```python
from build123d import *

# Parameters (mm, degrees)
SKETCH1_W           = 86.9
SKETCH1_H           = 86.9
BOSS_EXTRUDE1_DEPTH = 2
SKETCH2_R           = 1.65
CUT_EXTRUDE3_DEPTH  = 123.911431527
SKETCH3_W           = 18
SKETCH3_H           = 17
BOSS_EXTRUDE2_DEPTH = 1
SKETCH4_W           = 13
SKETCH4_H           = 14
CUT_EXTRUDE4_DEPTH  = 1
SKETCH5_R           = 15
CUT_EXTRUDE5_DEPTH  = 2


with BuildPart() as part:
    # Sketch1 → Boss-Extrude1 (new body)
    with BuildSketch(Plane(origin=(0, 0, 0), x_dir=(0, 1, 0), z_dir=(0, 0, 1))):
        with Locations((43.45, 43.45)):
            Rectangle(SKETCH1_W, SKETCH1_H)
    extrude(amount=BOSS_EXTRUDE1_DEPTH)

    # Sketch2 → Cut-Extrude3 (cut, through all)
    with BuildSketch(Plane.XY.offset(2)):
        with Locations((-84.05, 2.85)):
            Circle(SKETCH2_R)
        with Locations((-2.85, 2.85)):
            Circle(SKETCH2_R)
        with Locations((-2.85, 84.05)):
            Circle(SKETCH2_R)
        with Locations((-84.05, 84.05)):
            Circle(SKETCH2_R)
    extrude(amount=-CUT_EXTRUDE3_DEPTH, mode=Mode.SUBTRACT)

    # Sketch3 → Boss-Extrude2 (add)
    with BuildSketch(Plane.XY.offset(2)):
        with Locations((-63.4, 23.5)):
            Rectangle(SKETCH3_W, SKETCH3_H)
    extrude(amount=BOSS_EXTRUDE2_DEPTH)

    # Sketch4 → Cut-Extrude4 (cut)
    with BuildSketch(Plane.XY.offset(3)):
        with Locations((-63.4, 23.5)):
            Rectangle(SKETCH4_W, SKETCH4_H)
    extrude(amount=-CUT_EXTRUDE4_DEPTH, mode=Mode.SUBTRACT)

    # Sketch5 → Cut-Extrude5 (cut)
    with BuildSketch(Plane.XY.offset(2)):
        with Locations((-63.45, 63.45)):
            Circle(SKETCH5_R)
        with Locations((-23.45, 63.45)):
            Circle(SKETCH5_R)
        with Locations((-23.45, 23.45)):
            Circle(SKETCH5_R)
    extrude(amount=-CUT_EXTRUDE5_DEPTH, mode=Mode.SUBTRACT)


solid = part.part
```
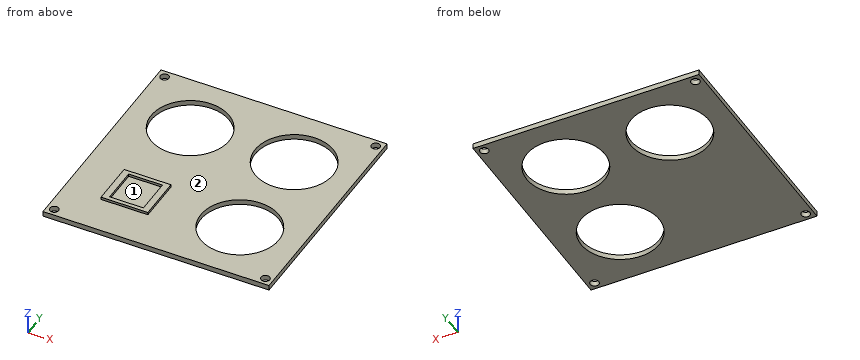
Check sheet for the modelled part. Datum: model origin and axes. Units: mm. Face numbers are marked on the shaded views. Give positions to 0.01 mm unless a question says otherwise; leave off trailing zeros. Order: outer loops, then holes, each group sorted by start corner. A loop starts at its lowest first (then second) coordinate and runs counter-clockwise, first axis right, second up. Notation, with made-up numbers: M -10,2.25 L 36,2.25 A31 cw 36,35.25 Z; hole C -32.5,-17 d6. An arc over 180 degrees is marked long. Answer in a Markdown table with one row per item. Add a question column.
Q1. Sectioned sample at D-D, the plane z = 2.5. Record the boundary of the cut face in (x, y), and give its area (3 significant figures).
Q2. Sectioned sample at B-B, the plane x = -2.85. Record the boundary of the cut face in (y, z).
Q3. Sectioned sample at A-A, the plane y = 84.05. Record the boundary of the cut face in (x, z).
Q4. Sectioned sample at C-C, the plane y = 23.45. Record the boundary of the cut face in (x, z), and give its area (3 significant figures).
Q5. Release check for a two-part mould opening along Y. For the marked faces 1 and 2 record: released by +Y, released by -Y, zero draft, split by the parting line, or undercut.
Q6. Thickness scan on L1, parallel to X at y = 84.05, z = 1.2; L2, parallel to Y at x = -84.05, z = 1.1; L3, parallel to X at y = 23, z = 1.5. Record the ranges inside material, lowest first.
Q7. Gauge pin test, flat ends, axial feed: pin 1 Ø2.5 at (x, y) = (-84.05, 84.05) entering from -Z; pin 2 Ø0.8 at (y, z) = (20, 2.5) entering from +X; pin 3 Ø0.5 at (x, z) = (-66, 2.5) entering from +Y; pin 4 Ø4 at (x, y) = (-60, 20) entering from +Z. Record the tip position at first contact, or that the pin passes through.
Verdict:
| question | item | result |
|---|---|---|
| 1 | outline | M -72.4,15 L -54.4,15 L -54.4,32 L -72.4,32 Z; hole M -69.9,16.5 L -56.9,16.5 L -56.9,30.5 L -69.9,30.5 Z |
| 1 | area | 124 mm² |
| 2 | outline | M 0,0 L 1.2,0 L 1.2,2 L 0,2 Z; M 4.5,0 L 82.4,0 L 82.4,2 L 4.5,2 Z; M 85.7,0 L 86.9,0 L 86.9,2 L 85.7,2 Z |
| 3 | outline | M -86.9,0 L -85.7,0 L -85.7,2 L -86.9,2 Z; M -82.4,0 L -4.5,0 L -4.5,2 L -82.4,2 Z; M -1.2,0 L 0,0 L 0,2 L -1.2,2 Z |
| 4 | outline | M -86.9,0 L -38.45,0 L -38.45,2 L -54.4,2 L -54.4,3 L -56.9,3 L -56.9,2 L -69.9,2 L -69.9,3 L -72.4,3 L -72.4,2 L -86.9,2 Z; M -8.45,0 L 0,0 L 0,2 L -8.45,2 Z |
| 4 | area | 119 mm² |
| 5 | face 1 | undercut |
| 5 | face 2 | zero draft |
| 6 | L1 | -86.9 to -85.7, -82.4 to -4.5, -1.2 to 0 |
| 6 | L2 | 0 to 1.2, 4.5 to 82.4, 85.7 to 86.9 |
| 6 | L3 | -86.9 to -38.44, -8.46 to 0 |
| 7 | pin 1 | through |
| 7 | pin 2 | x = -54.4 |
| 7 | pin 3 | y = 32 |
| 7 | pin 4 | z = 2 |
